```python
from build123d import *

# Parameters (mm, degrees)
ESQUISSE1_W             = 340
ESQUISSE1_H             = 165
BOSS_EXTRU_1_DEPTH      = 6
ESQUISSE2_W             = 6
ESQUISSE2_H             = 35
ESQUISSE2_H_2           = 20
ESQUISSE2_W_2           = 68
ESQUISSE2_H_3           = 6
ESQUISSE2_H_4           = 25
ESQUISSE2_W_3           = 40
ESQUISSE2_H_5           = 50
ESQUISSE2_W_4           = 20
ENL_V_MAT_EXTRU_1_DEPTH = 6
ESQUISSE3_W             = 6
ESQUISSE3_H             = 20
ESQUISSE3_W_2           = 20
ESQUISSE3_H_2           = 6
ESQUISSE3_W_3           = 30
ESQUISSE3_H_3           = 15
ENL_V_MAT_EXTRU_2_DEPTH = 10
ESQUISSE5_R             = 1.5
ESQUISSE5_W             = 10
ESQUISSE5_H             = 6
ENL_V_MAT_EXTRU_4_DEPTH = 6
ESQUISSE7_R             = 1.5
ESQUISSE7_R_2           = 1.505
ESQUISSE7_W             = 10
ESQUISSE7_H             = 15
ENL_V_MAT_EXTRU_7_DEPTH = 378.969575495
ESQUISSE8_R             = 2.995
ESQUISSE8_R_2           = 3
ENL_V_MAT_EXTRU_9_DEPTH = 3


with BuildPart() as part:
    # Esquisse1 → Boss.-Extru.1 (new body)
    with BuildSketch(Plane.XY):
        with Locations((-170, 82.5)):
            Rectangle(ESQUISSE1_W, ESQUISSE1_H)
    extrude(amount=BOSS_EXTRU_1_DEPTH)

    # Esquisse2 → Enlèv. mat.-Extru.1 (cut)
    with BuildSketch(Plane.XY.offset(6)):
        Polygon((0, 165), (0, 135), (-6, 135), (-6, 159), (-35, 159), (-35, 165), align=None)
        Polygon((-340, 165), (-272, 165), (-272, 159), (-334, 159), (-334, 120), (-340, 120), align=None)
        with Locations((-337, 82.5)):
            Rectangle(ESQUISSE2_W, ESQUISSE2_H)
        with Locations((-67, 102)):
            Rectangle(ESQUISSE2_W, ESQUISSE2_H_2)
        with Locations((-170, 162)):
            Rectangle(ESQUISSE2_W_2, ESQUISSE2_H_3)
        with Locations((-3, 12.5)):
            Rectangle(ESQUISSE2_W, ESQUISSE2_H_4)
        with Locations((-337, 17.5)):
            Rectangle(ESQUISSE2_W, ESQUISSE2_H)
        with Locations((-84, 162)):
            Rectangle(ESQUISSE2_W_3, ESQUISSE2_H_3)
        with Locations((-3, 80)):
            Rectangle(ESQUISSE2_W, ESQUISSE2_H_5)
        with Locations((-36, 58)):
            Rectangle(ESQUISSE2_W_4, ESQUISSE2_H_3)
    extrude(amount=-ENL_V_MAT_EXTRU_1_DEPTH, mode=Mode.SUBTRACT)

    # Esquisse3 → Enlèv. mat.-Extru.2 (cut)
    with BuildSketch(Plane(origin=(0, 0, 0), x_dir=(-1, 0, 0), z_dir=(0, 0, -1))):
        with Locations((241, 119)):
            Rectangle(ESQUISSE3_W, ESQUISSE3_H)
        with Locations((241, 59)):
            Rectangle(ESQUISSE3_W, ESQUISSE3_H)
        with Locations((288.5, 87.5)):
            Rectangle(ESQUISSE3_W, ESQUISSE3_H)
        with Locations((310, 48.5)):
            Rectangle(ESQUISSE3_W_2, ESQUISSE3_H_2)
        with Locations((319, 151.5)):
            Rectangle(ESQUISSE3_W_3, ESQUISSE3_H_3)
    extrude(amount=-ENL_V_MAT_EXTRU_2_DEPTH, mode=Mode.SUBTRACT)

    # Esquisse5 → Enlèv. mat.-Extru.4 (cut)
    with BuildSketch(Plane(origin=(0, 0, 0), x_dir=(-1, 0, 0), z_dir=(0, 0, -1))):
        with Locations((151.5, 136)):
            Circle(ESQUISSE5_R)
        with Locations((151.5, 24)):
            Circle(ESQUISSE5_R)
        with Locations((134, 136)):
            Rectangle(ESQUISSE5_W, ESQUISSE5_H)
        with Locations((169, 136)):
            Rectangle(ESQUISSE5_W, ESQUISSE5_H)
        with Locations((134, 24)):
            Rectangle(ESQUISSE5_W, ESQUISSE5_H)
        with Locations((169, 24)):
            Rectangle(ESQUISSE5_W, ESQUISSE5_H)
    extrude(amount=-ENL_V_MAT_EXTRU_4_DEPTH, mode=Mode.SUBTRACT)

    # Esquisse7 → Enlèv. mat.-Extru.7 (cut, through all)
    with BuildSketch(Plane(origin=(0, 0, 0), x_dir=(-1, 0, 0), z_dir=(0, 0, -1))):
        with Locations((337, 50)):
            Circle(ESQUISSE7_R)
        with Locations((319.5, 140)):
            Circle(ESQUISSE7_R)
        with Locations((42, 162)):
            Circle(ESQUISSE7_R)
        with Locations((293, 48.5)):
            Circle(ESQUISSE7_R)
        with Locations((327, 48.5)):
            Circle(ESQUISSE7_R)
        with Locations((288.5, 70.5)):
            Circle(ESQUISSE7_R)
        with Locations((288.5, 104.5)):
            Circle(ESQUISSE7_R)
        with Locations((241, 39)):
            Circle(ESQUISSE7_R)
        with Locations((241, 79)):
            Circle(ESQUISSE7_R)
        with Locations((241, 99)):
            Circle(ESQUISSE7_R)
        with Locations((241, 139)):
            Circle(ESQUISSE7_R)
        with Locations((241, 7)):
            Circle(ESQUISSE7_R)
        with Locations((57, 162)):
            Circle(ESQUISSE7_R)
        with Locations((262, 162)):
            Circle(ESQUISSE7_R)
        with Locations((214, 162)):
            Circle(ESQUISSE7_R)
        with Locations((111, 162)):
            Circle(ESQUISSE7_R)
        with Locations((138, 162)):
            Circle(ESQUISSE7_R)
        with Locations((129, 162)):
            Circle(ESQUISSE7_R)
        with Locations((67, 85)):
            Circle(ESQUISSE7_R)
        with Locations((67, 119)):
            Circle(ESQUISSE7_R)
        with Locations((53, 58)):
            Circle(ESQUISSE7_R)
        with Locations((19, 58)):
            Circle(ESQUISSE7_R)
        with Locations((3, 32)):
            Circle(ESQUISSE7_R_2)
        with Locations((3, 48)):
            Circle(ESQUISSE7_R)
        with Locations((3, 112)):
            Circle(ESQUISSE7_R)
        with Locations((3, 128)):
            Circle(ESQUISSE7_R)
        with Locations((337, 110)):
            Circle(ESQUISSE7_R)
        with Locations((329, 7.5)):
            Rectangle(ESQUISSE7_W, ESQUISSE7_H)
    extrude(amount=-ENL_V_MAT_EXTRU_7_DEPTH, mode=Mode.SUBTRACT)

    # Esquisse8 → Enlèv. mat.-Extru.9 (cut)
    with BuildSketch(Plane(origin=(0, 0, 0), x_dir=(-1, 0, 0), z_dir=(0, 0, -1))):
        with Locations((3, 32)):
            Circle(ESQUISSE8_R)
        with Locations((3, 48)):
            Circle(ESQUISSE8_R)
        with Locations((19, 58)):
            Circle(ESQUISSE8_R_2)
        with Locations((3, 112)):
            Circle(ESQUISSE8_R)
        with Locations((3, 128)):
            Circle(ESQUISSE8_R)
        with Locations((53, 58)):
            Circle(ESQUISSE8_R_2)
        with Locations((67, 85)):
            Circle(ESQUISSE8_R_2)
        with Locations((67, 119)):
            Circle(ESQUISSE8_R_2)
        with Locations((111, 162)):
            Circle(ESQUISSE8_R)
        with Locations((42, 162)):
            Circle(ESQUISSE8_R)
        with Locations((129, 162)):
            Circle(ESQUISSE8_R)
        with Locations((151.5, 136)):
            Circle(ESQUISSE8_R_2)
        with Locations((151.5, 24)):
            Circle(ESQUISSE8_R_2)
        with Locations((214, 162)):
            Circle(ESQUISSE8_R)
        with Locations((57, 162)):
            Circle(ESQUISSE8_R)
        with Locations((262, 162)):
            Circle(ESQUISSE8_R)
        with Locations((241, 139)):
            Circle(ESQUISSE8_R_2)
        with Locations((241, 99)):
            Circle(ESQUISSE8_R_2)
        with Locations((241, 79)):
            Circle(ESQUISSE8_R_2)
        with Locations((241, 39)):
            Circle(ESQUISSE8_R_2)
        with Locations((241, 7)):
            Circle(ESQUISSE8_R_2)
        with Locations((337, 50)):
            Circle(ESQUISSE8_R)
        with Locations((327, 48.5)):
            Circle(ESQUISSE8_R_2)
        with Locations((293, 48.5)):
            Circle(ESQUISSE8_R_2)
        with Locations((288.5, 70.5)):
            Circle(ESQUISSE8_R_2)
        with Locations((288.5, 104.5)):
            Circle(ESQUISSE8_R_2)
        with Locations((319.5, 140)):
            Circle(ESQUISSE8_R)
        with Locations((337, 110)):
            Circle(ESQUISSE8_R)
    extrude(amount=-ENL_V_MAT_EXTRU_9_DEPTH, mode=Mode.SUBTRACT)


solid = part.part
```
Check sheet for the modelled part. Datum: model origin and axes. Units: mm. A direction names the side the tool comes from. Give positions to 0.01 mm unless a question says otherwise; leave off trailing zeros. Order: outer loops, then holes, each group sorted by start corner. A loop starts at its lowest first (then second) coordinate and runs counter-clockwise, first axis right, second up. Notation, with made-up numbers: M 19,17.5 L 38,17.5 A25 cw 38,33.5 Z; hole C 15,33.5 d6. An arc over 180 degrees is marked long. Answer in a Markdown table with one row per item. Add a question column.
Q1. Thickness scan on L1, parallel to Y at x = -67, z = 2.15; L2, parallel to Y at x = -288.5, z = 1.7; L3, parallel to Y at x = -168, z = 1.95. Record the ranges inside material, lowest first.
Q2. Sectioned sample at B-B, the plane x = -30.5. Record the boundary of the cut face in (y, z).
Q3. Sectioned sample at C-C, the plane z = 1.55. Count the separate pieces of the cut face and the enclosed holes in it, and give its area (3 significant figures).
Q4. Sectioned sample at A-A, the plane x = -170.5. Record the boundary of the cut face in (y, z), and give its area (3 significant figures).
Q5. Gauge pin test, flat ends, axial feed: pin 1 Ø5.5 at (x, y) = (-241, 39) entering from -Z; pin 2 Ø3 at (y, z) = (135.5, 4) entering from -X; pin 3 Ø3 at (y, z) = (150, 2) entering from -X. Record the tip position at first contact, or that the pin passes through.
Q6. Access from +Z, -Z, +X, -X, +Y, -Y to the whole of each face (thin tool, end or side, straight path). Record for faces 4 (the flat face through (-150, 135, 3)), 5 (the flat face through (-304, 151, 3)), 6 (the flat face through (-129, 24, 3)).
Q7. Release check for a two-part mould opening along Y. For faces 1 (the cylindrical face through (-110.351, 159.076, 1.479)), 2 (the flat face through (-172, 84, 6)), 3 (the flat face through (-84, 159, 3)) record: released by +Y, released by -Y, zero draft, split by the parting line, or undercut.
Q8. Sectioned sample at D-D, the plane y = 154. Record the boundary of the cut face in (x, z), and give its area (3 significant figures).
Verdict:
| question | item | result |
|---|---|---|
| 1 | L1 | 0 to 82, 88 to 92, 112 to 116, 122 to 159 |
| 1 | L2 | 0 to 67.5, 73.5 to 77.5, 97.5 to 101.5, 107.5 to 159 |
| 1 | L3 | 0 to 21, 27 to 133, 139 to 159 |
| 2 | outline | M 0,0 L 55,0 L 55,6 L 0,6 Z; M 61,0 L 159,0 L 159,6 L 61,6 Z |
| 3 | separate pieces | 1 |
| 3 | enclosed holes | 38 |
| 3 | area | 51,200 mm² |
| 4 | outline | M 0,0 L 21,0 L 21,6 L 0,6 Z; M 27,0 L 133,0 L 133,6 L 27,6 Z; M 139,0 L 159,0 L 159,6 L 139,6 Z |
| 4 | area | 882 mm² |
| 5 | pin 1 | z = 3 |
| 5 | pin 2 | x = -334 |
| 5 | pin 3 | x = -304 |
| 6 | face 4 | -Z |
| 6 | face 5 | +Z, -Z, -X, +Y |
| 6 | face 6 | +Z, -Z |
| 7 | face 1 | undercut |
| 7 | face 2 | zero draft |
| 7 | face 3 | released by +Y |
| 8 | outline | M -304,0 L -6,0 L -6,6 L -304,6 Z |
| 8 | area | 1,790 mm² |
